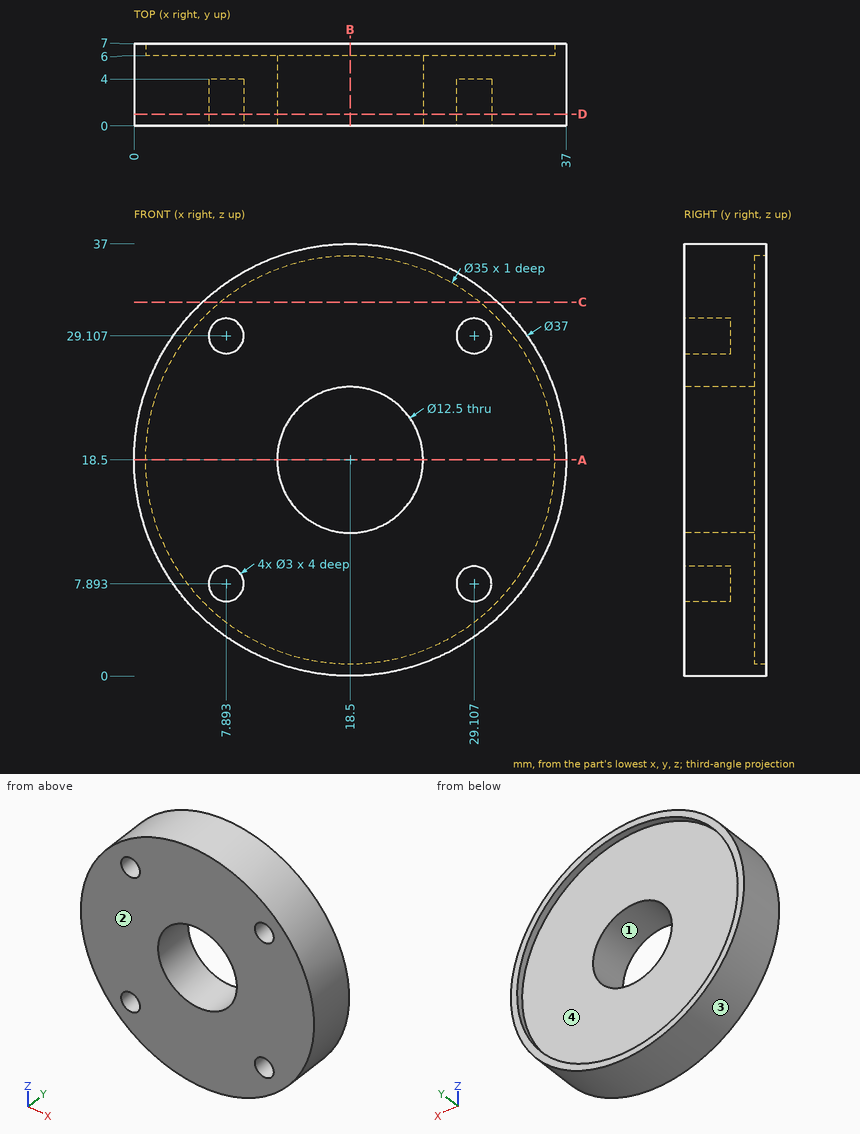
Here's the drawing with two shaded views (mm, measured from the low corner). I have some questions. Round coordinates to 2 decimals unless told otherwise and drop trailing zeros. Order: outer loops, then holes, each group sorted by start corner. A loop starts at its lowest first (then second) coordinate and runs counter-clockwise, first axis right, second up. Notation, with made-up numbers: (39, -4.75) -> (47, -4.75) arc R20 ccw to (47, 26.25) -> close; hole circle Ø9 at (0, 21.5). An arc over 180 degrees is marked (long way). Return JSON: item names as keys, results as strings.
Q1. If we mould it in two halves opening along X, with no side actions, what happens to the marked faces 1, 2, 3 and 4? For each: released by +X, released by -X, zero draft, split by the parting line, or undercut.
Filled sheet:
{"face 1": "undercut", "face 2": "zero draft", "face 3": "split by the parting line", "face 4": "undercut"}
Q2. For pin 1 Ø1.8 at (x, z) = (29.11, 7.89) entering from -Y; pin 2 Ø1.5 at (y, z) = (3, 30.5) entering from -X (1 decimal); pin 3 Ø3 at (y, z) = (1, 9.5) entering from +X, each with a flat end and sliding along its axis, tell me the tip position at first contact or that it passes through.
Filled sheet:
{"pin 1": "stops at y = 4", "pin 2": "stops at x = 3.8", "pin 3": "stops at x = 35.41"}
Q3. If we section it at A-A on z = 18.5: List the corners of the cut face in (x, y) for me, plus the area to 3 significant figures.
Filled sheet:
{"outline": "(0, 0) -> (12.25, 0) -> (12.25, 6) -> (1, 6) -> (1, 7) -> (0, 7) -> close; (24.75, 0) -> (37, 0) -> (37, 7) -> (36, 7) -> (36, 6) -> (24.75, 6) -> close", "area": "149 mm^2"}
Q4. If we section it at B-B on x = 18.5: List the corners of the cut face in (y, z) for me.
Filled sheet:
{"outline": "(0, 0) -> (7, 0) -> (7, 1) -> (6, 1) -> (6, 12.25) -> (0, 12.25) -> close; (0, 24.75) -> (6, 24.75) -> (6, 36) -> (7, 36) -> (7, 37) -> (0, 37) -> close"}
Q5. If we section it at C-C on z = 32: List the corners of the cut face in (x, y) for me (1 decimal).
Filled sheet:
{"outline": "(5.9, 0) -> (31.1, 0) -> (31.1, 7) -> (29.6, 7) -> (29.6, 6) -> (7.4, 6) -> (7.4, 7) -> (5.9, 7) -> close"}
Q6. I need wall thicknesses on line 1 along Z through (x, y) = (7, 1.5); line 2 along Z through (x, y) = (7.5, 2.5) (1 decimal); line 3 along X through (y, z) = (1.25, 9) (1 decimal). Which ranges of each line are inside material? Lowest first, please. Write a range as from..to.
Filled sheet:
{"line 1": "z = 4.01..6.69, 9.1..27.9, 30.31..32.99", "line 2": "z = 3.6..6.4, 9.3..27.7, 30.6..33.4", "line 3": "x = 2.6..6.9, 8.9..28.1, 30.1..34.4"}
Q7. If we section it at D-D on y = 1: List the corners of the cut face in (x, z) for me, plus the area to 3 significant figures.
Filled sheet:
{"outline": "circle Ø37 at (18.5, 18.5); hole circle Ø3 at (7.89, 7.89); hole circle Ø3 at (7.89, 29.11); hole circle Ø12.5 at (18.5, 18.5); hole circle Ø3 at (29.11, 7.89); hole circle Ø3 at (29.11, 29.11)", "area": "924 mm^2"}
